Check sheet for the modelled part. Datum: model origin and axes. Units: mm. A direction names the side the tool comes from. Round coordinates to 2 decimals unless told otherwise and drop trailing zeros. Loops run counter-clockwise (first coordinate to the right, second up) from the corner with the lowest first, then second, coordinate; pieces in that order, holes last. Notation, with made-up numbers: (15, -13.5) -> (19, -13.5) arc R14 cw to (19, 13.5) -> close; hole circle Ø2 at (39, -22). An arc over 180 degrees is marked (long way). Use one line per item in the form item = value. Start each with the question number.
(1) Sectioned sample at B-B (x = 78). Record the cut outline in (y, z), and give its area (3 significant figures).
(2) Material ranges on probe 1 along Y at (x, z) = (64.25, 4.5); probe 2 along Y at (x, z) = (64.5, 3.2); probe 3 along Y at (x, z) = (64.5, 4.3), recorded low to high. Write a range as [from, to].
(3) Go/stop test with flat-tipped pins: pin 1 (6 mm diameter, centred on x = 68.5, y = -4, fed in from -Z); pin 2 (2.5 mm diameter, centred on x = 78.27, y = 19.74, fed in from +Z); pin 3 (3 mm diameter, centred on y = 17, z = 1.5, fed in from -X); pin 4 (4 mm diameter, centred on x = 54.27, y = 19.74, fed in from +Z). Record where each tip stops, or that it passes through.
(4) Sectioned sample at A-A (y = -11.5). Record the cut outline in (x, z), and give its area (3 significant figures).
(5) Set-up check for faces 1 (the cylindrical face through (66.25, 4.21, 2.43)), 2 (the cylindrical face through (53.17, -11.24, 4.68)): record each of +Z, -Z, +X, -X, +Y, -Y from which the full face is reachable in a straight line by a thin tool's end or side.
(6) Draft check along Y on faces 3 (the cylindrical face through (66.25, 14.81, 2.43)), 4 (the cylindrical face through (77.17, -11.24, 4.68)), 5 (the flat face through (51.773, 3, 5)), 6 (the flat face through (66, -14.756, 5)). Enter one of: released by +Y, released by -Y, zero draft, split by the parting line, or undercut.
(7) Sectioned sample at C-C (z = 4.4). Record the cut outline in (x, y), and give its area (3 significant figures).
(8) Sectioned sample at D-D (z = 1.9). Record the cut outline in (x, y), and give its area (3 significant figures).
from build123d import *

# Parameters (mm, degrees)
SKETCH2_W           = 19
SKETCH2_H           = 27
SKETCH2_R           = 3.5
BOSS_EXTRUDE1_DEPTH = 2
SKETCH3_R           = 3.5
SKETCH3_R_2         = 2.5
BOSS_EXTRUDE2_DEPTH = 5
FILLET1_R           = 0.5
SKETCH6_W           = 29
SKETCH6_H           = 37
SKETCH6_R           = 1.5
SKETCH6_W_2         = 19
SKETCH6_H_2         = 27
BOSS_EXTRUDE6_DEPTH = 2


with BuildPart() as part:
    # Sketch2 → Boss-Extrude1 (new body)
    with BuildSketch(Plane(origin=(0, 0, 5.662636572), x_dir=(-1, 0, 0), z_dir=(0, 0, -1))):
        with Locations((-66.272536925, 3.74415348)):
            Rectangle(SKETCH2_W, SKETCH2_H)
        with Locations((-63.672536925, 12.44415348)):
            Circle(SKETCH2_R, mode=Mode.SUBTRACT)
        with Locations((-63.672536925, 1.84415348)):
            Circle(SKETCH2_R, mode=Mode.SUBTRACT)
    extrude(amount=BOSS_EXTRUDE1_DEPTH)

    # Sketch3 → Boss-Extrude2 (add)
    # profile 1 of 2: a face of its own
    with BuildSketch(Plane(origin=(0, 0, 5.662636572), x_dir=(-1, 0, 0), z_dir=(0, 0, -1))):
        with Locations((-63.672536925, 12.44415348)):
            Circle(SKETCH3_R)
        with Locations((-63.672536925, 12.44415348)):
            Circle(SKETCH3_R_2, mode=Mode.SUBTRACT)
    # profile 2 of 2: a face of its own
    with BuildSketch(Plane(origin=(0, 0, 5.662636572), x_dir=(-1, 0, 0), z_dir=(0, 0, -1))):
        with Locations((-63.672536925, 1.84415348)):
            Circle(SKETCH3_R)
        with Locations((-63.672536925, 1.84415348)):
            Circle(SKETCH3_R_2, mode=Mode.SUBTRACT)
    extrude(amount=BOSS_EXTRUDE2_DEPTH)

    # Fillet1
    fillet1_edges = [part.edges().sort_by_distance(p)[0] for p in [
        (67.172536925, 12.44415348, 0.662636572),
        (67.172536925, 1.84415348, 0.662636572),
    ]]
    fillet(fillet1_edges, radius=FILLET1_R)

    # Sketch6 → Boss-Extrude6 (add)
    with BuildSketch(Plane.XY.offset(5.662636572)):
        with Locations((66.272536925, 3.74415348)):
            Rectangle(SKETCH6_W, SKETCH6_H)
        with Locations((54.272536925, 19.74415348)):
            Circle(SKETCH6_R, mode=Mode.SUBTRACT)
        with Locations((78.272536925, 19.74415348)):
            Circle(SKETCH6_R, mode=Mode.SUBTRACT)
        with Locations((78.272536925, -12.25584652)):
            Circle(SKETCH6_R, mode=Mode.SUBTRACT)
        with Locations((54.272536925, -12.25584652)):
            Circle(SKETCH6_R, mode=Mode.SUBTRACT)
        with Locations((66.272536925, 3.74415348)):
            Rectangle(SKETCH6_W_2, SKETCH6_H_2, mode=Mode.SUBTRACT)
    extrude(amount=-BOSS_EXTRUDE6_DEPTH)


solid = part.part
Checks:
q1.outline = (-14.76, 3.66) -> (-13.73, 3.66) -> (-13.73, 5.66) -> (-14.76, 5.66) -> close; (-10.78, 3.66) -> (18.27, 3.66) -> (18.27, 5.66) -> (-10.78, 5.66) -> close; (21.22, 3.66) -> (22.24, 3.66) -> (22.24, 5.66) -> (21.22, 5.66) -> close
q1.area = 62.2 mm2
q2.probe_1 = [-14.76, -0.59], [4.28, 10.01], [14.88, 22.24]
q2.probe_2 = [-1.56, -0.51], [4.2, 5.24], [9.04, 10.09], [14.8, 15.84]
q2.probe_3 = [-14.76, -0.51], [4.2, 10.09], [14.8, 22.24]
q3.pin_1 = 3.66
q3.pin_2 = through
q3.pin_3 = 61.97
q3.pin_4 = 5.66
q4.outline = (51.77, 3.66) -> (52.98, 3.66) -> (52.98, 5.66) -> (51.77, 5.66) -> close; (55.57, 3.66) -> (76.98, 3.66) -> (76.98, 5.66) -> (55.57, 5.66) -> close; (79.57, 3.66) -> (80.77, 3.66) -> (80.77, 5.66) -> (79.57, 5.66) -> close
q4.area = 47.6 mm2
q5.face_1 = -Z
q5.face_2 = +Z, -Z
q6.face_3 = undercut
q6.face_4 = undercut
q6.face_5 = zero draft
q6.face_6 = released by -Y
q7.outline = (51.77, -14.76) -> (80.77, -14.76) -> (80.77, 22.24) -> (51.77, 22.24) -> close; hole circle Ø3 at (54.27, -12.26); hole circle Ø3 at (54.27, 19.74); hole circle Ø5 at (63.67, 1.84); hole circle Ø5 at (63.67, 12.44); hole circle Ø3 at (78.27, -12.26); hole circle Ø3 at (78.27, 19.74)
q7.area = 1,010 mm2
q8.outline = circle Ø7 at (63.67, 1.84); circle Ø7 at (63.67, 12.44); hole circle Ø5 at (63.67, 1.84); hole circle Ø5 at (63.67, 12.44)
q8.area = 37.7 mm2
